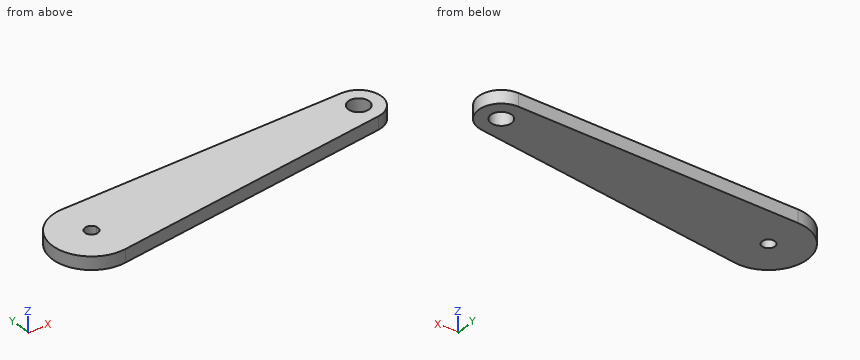
```python
from build123d import *

# Parameters (mm, degrees)
SKETCH_2_R          = 15
SKETCH_2_R_2        = 8.75
EXTRUDE_1_DEPTH     = 5
SKETCH_3_R          = 4
CUT_EXTRUDE_1_DEPTH = 5


with BuildPart() as part:
    # 草图2 → 凸台-拉伸1 (new body)
    with BuildSketch(Plane.XY):
        Circle(SKETCH_2_R)
        with BuildLine():
            Line((108.957293046, 15.310277664), (-0.042706954, 14.999939204))
            ThreePointArc((-0.042706954, 14.999939204), (10.591491767, 10.621690174), (15, 0))
            ThreePointArc((15, 0), (11.210584144, -9.966082639), (1.756959578, -14.896747734))
            Line((1.756959578, -14.896747734), (110.007098523, -2.129456383))
            ThreePointArc((110.007098523, -2.129456383), (100.248015648, 6.034548214), (108.957293046, 15.310277664))
        make_face()
        with Locations((108.982205436, 6.560313128)):
            Circle(SKETCH_2_R_2)
    extrude(amount=EXTRUDE_1_DEPTH)

    # 草图3 → 切除-拉伸1 (cut)
    with BuildSketch(Plane.XY.offset(5)):
        with BuildLine():
            Line((2.4, -0.7), (2.4, 0))
            Line((2.4, 0), (2.4, 0.7))
            ThreePointArc((2.4, 0.7), (-2.5, 0), (2.4, -0.7))
        make_face()
        with Locations((108.982205436, 6.560313128)):
            Circle(SKETCH_3_R)
    extrude(amount=-CUT_EXTRUDE_1_DEPTH, mode=Mode.SUBTRACT)


solid = part.part
```
Design review of the part built by this model. Coordinates are the model's own, in mm. Give positions to 0.01 mm unless a question says otherwise; leave off trailing zeros. Write each loop counter-clockwise with the first axis right and the second up, starting at its lowest first coordinate (ties: lowest second). Pieces come first, ordered by that corner, then holes.
(1) Add section C-C (x = 18). Give the boundary of the cut face in (y, z), and give its area (3 significant figures).
Checked values:
outline: (-12.98, 0) - (15.05, 0) - (15.05, 5) - (-12.98, 5) - close
area: 140 mm2
(2) Add section B-B (z = 3.3). Give the boundary of the cut face in (x, y).
Checked values:
outline: (-0.04, 15) arc R15 ccw (long way) to (1.76, -14.9) - (110.01, -2.13) arc R8.75 ccw to (108.96, 15.31) - close; hole (2.4, -0.7) - (2.4, 0.7) arc R2.5 ccw (long way) to start; hole circle Ø8 at (108.98, 6.56)
(3) Add section D-D (y = -12). Give the boundary of the cut face in (x, z).
Checked values:
outline: (-9, 0) - (26.32, 0) - (26.32, 5) - (-9, 5) - close
(4) Wall thickness on line 1 along Y through (x, z) = (0, 3.7); line 2 along Y through (x, z) = (-1, 3.25); line 3 along X through (y, z) = (3, 0.8): over which ranges is each line inside the solid? List them lowest first.
Checked values:
line 1: y = -15 to -2.5, 2.5 to 15
line 2: y = -14.97 to -2.29, 2.29 to 14.97
line 3: x = -14.7 to 107.16, 110.81 to 116.98
(5) Clearance check with flat-ended pins moving along their axes: pin 1 Ø1.5 at (y, z) = (0.5, 3) entering from -X; pin 2 Ø3 at (y, z) = (7, 4.5) entering from -X; pin 3 Ø1 at (x, z) = (65.5, 4) entering from +Y. State where each tip first meets the part, or that it passes through.
Checked values:
pin 1: stops at x = -15
pin 2: stops at x = -13.96
pin 3: stops at y = 15.19
(6) Add section A-A (y = 5). Give the boundary of the cut face in (x, z), and give its area (3 significant figures).
Checked values:
outline: (-14.14, 0) - (105.3, 0) - (105.3, 5) - (-14.14, 5) - close; (112.67, 0) - (117.59, 0) - (117.59, 5) - (112.67, 5) - close
area: 622 mm2
